```python
from build123d import *

# Parameters (mm, degrees)
SKETCH1_R           = 1.7859375
BOSS_EXTRUDE1_DEPTH = 0.8128


with BuildPart() as part:
    # Sketch1 → Boss-Extrude1 (new body)
    with BuildSketch(Plane.XY):
        with BuildLine():
            Line((2.778125, 0), (13.824739587, 0))
            ThreePointArc((13.824739587, 0), (15.795261881, -0.592725305), (17.111798004, -2.174184768))
            ThreePointArc((17.111798004, -2.174184768), (20.879142703, -5.390786788), (25.716280165, -4.322369358))
            ThreePointArc((25.716280165, -4.322369358), (27.621647146, -3.545286331), (29.639532121, -3.948301955))
            ThreePointArc((29.639532121, -3.948301955), (33.02176359, -3.935123977), (34.876672666, -1.106877933))
            ThreePointArc((34.876672666, -1.106877933), (31.588422177, 8.579995637), (22.225, 12.7))
            Line((22.225, 12.7), (15.08125, 12.7))
            ThreePointArc((15.08125, 12.7), (12.555552966, 11.653822034), (11.509375, 9.128125))
            ThreePointArc((11.509375, 9.128125), (10.463197034, 6.602427966), (7.9375, 5.55625))
            Line((7.9375, 5.55625), (0.813693974, 5.55625))
            ThreePointArc((0.813693974, 5.55625), (0.238325447, 5.317924553), (0, 4.742556026))
            Line((0, 4.742556026), (0, 2.778125))
            ThreePointArc((0, 2.778125), (0.813693974, 0.813693974), (2.778125, 0))
        make_face()
        with BuildLine():
            ThreePointArc((33.097531197, -0.951223224), (31.162735019, -2.574709983), (29.53924826, -0.639913805))
            ThreePointArc((29.53924826, -0.639913805), (27.638228446, 4.960309977), (22.225, 7.3421875))
            ThreePointArc((22.225, 7.3421875), (20.4390625, 9.128125), (22.225, 10.9140625))
            ThreePointArc((22.225, 10.9140625), (30.271690934, 7.37343375), (33.097531197, -0.951223224))
        make_face(mode=Mode.SUBTRACT)
        with Locations((22.225, 0)):
            Circle(SKETCH1_R, mode=Mode.SUBTRACT)
        with Locations((15.08125, 9.128125)):
            Circle(SKETCH1_R, mode=Mode.SUBTRACT)
    extrude(amount=BOSS_EXTRUDE1_DEPTH)


solid = part.part
```
CAD build for the part. Positions are in the model's coordinates, mm. A direction names the side the tool comes from. Give positions to 0.01 mm unless a question says otherwise; leave off trailing zeros. Write each loop counter-clockwise with the first axis right and the second up, starting at its lowest first coordinate (ties: lowest second). Pieces come first, ordered by that corner, then holes. Notation, with made-up numbers: M 48,56 L 106,56 A18 ccw 106,60 Z; hole C 24.5,-17.75 d11. An arc over 180 degrees is marked long. Return JSON: item names as keys, results as strings. Group by question number.
(1) 3-axis set-ups, long thin cutter, end or side, ignore diameter. For faces 4 (the face through (0.79, 0.84, 0.4)), 5 (the face through (4.4, 5.556, 0.4)), 6 (the face through (27.695, 4.897, 0.401)): which of +Z, -Z, +X, -X, +Y, -Y reach the whole face in a straight line?
(2) Drill centre lines: L1, parallel to X at y = 10, z = 0.55; L2, parallel to X at y = 8, z = 0.4; L3, parallel to X at y = 5, z = 0.55. Where is each one in solid material? Low to high. Write a range as [from, to].
(3) Band-saw the part on D-D (z = 0.25). Give the cut face in (x, y) (1 decimal).
(4) Flat gauge pin, fed straight in: pin 1 Ø6 at (x, y) = (14, -3.5) entering from +Z. Where does the tip first touch, or does it go through?
(5) Band-saw the part on C-C (y = 6). Give the cut face in (x, z).
(6) Band-saw the part on B-B (y = 0.5). Give the cut face in (x, z), and give its area (3 significant figures).
(7) Band-saw the part on A-A (x = 23). Give the cut face in (y, z), and give its area (3 significant figures).
(8) Mould opens along Y. For faces 1 (the face through (23.875, -0.684, 0.401)), 2 (the face through (8.2, 0, 0.4)), 3 (the face through (17, 4, 0.813)) say: pulls with the +Y half, pulls with the -Y half, needs draft (parallel to the pull), parting line crosses it, or undercut.
Entries:
{
 "1": {"face 4": "+Z, -Z, -X, -Y", "face 5": "+Z, -Z, -X, +Y", "face 6": "+Z, -Z"},
 "2": {"L1": "x = [11.62, 13.52], [16.64, 20.67], [26.6, 30.05]", "L2": "x = [11.33, 13.7], [16.47, 20.84], [29.65, 32.09]", "L3": "x = [0.04, 27.6], [31.93, 33.9]"},
 "3": {"outline": "M 0,2.8 A2.8 ccw 2.8,0 L 13.8,0 A3.6 cw 17.1,-2.2 A5.6 ccw 25.7,-4.3 A3.6 cw 29.6,-3.9 A3.6 ccw 34.9,-1.1 A12.7 ccw 22.2,12.7 L 15.1,12.7 A3.6 ccw 11.5,9.1 A3.6 cw 7.9,5.6 L 0.8,5.6 A0.8 ccw 0,4.7 Z; hole C 15.1,9.1 d3.6; hole C 22.2,0 d3.6; hole M 22.2,7.3 A7.3 cw 29.5,-0.6 A1.8 ccw 33.1,-1 A10.9 ccw 22.2,10.9 A1.8 ccw Z"},
 "4": {"pin 1": "passes through"},
 "5": {"outline": "M 9.66,0 L 26.46,0 L 26.46,0.81 L 9.66,0.81 Z; M 31.34,0 L 33.42,0 L 33.42,0.81 L 31.34,0.81 Z"},
 "6": {"outline": "M 1.19,0 L 20.51,0 L 20.51,0.81 L 1.19,0.81 Z; M 23.94,0 L 29.55,0 L 29.55,0.81 L 23.94,0.81 Z; M 33.13,0 L 34.92,0 L 34.92,0.81 L 33.13,0.81 Z", "area": "21.7 mm^2"},
 "7": {"outline": "M -5.5,0 L -1.61,0 L -1.61,0.81 L -5.5,0.81 Z; M 1.61,0 L 7.3,0 L 7.3,0.81 L 1.61,0.81 Z; M 10.89,0 L 12.68,0 L 12.68,0.81 L 10.89,0.81 Z", "area": "9.25 mm^2"},
 "8": {"face 1": "undercut", "face 2": "pulls with the -Y half", "face 3": "needs draft"}
}
